```python
from build123d import *

# Parameters (mm, degrees)
SKETCH1_W           = 38.1
SKETCH1_H           = 300
BOSS_EXTRUDE1_DEPTH = 5
SKETCH4_W           = 9
SKETCH4_H           = 40
BOSS_EXTRUDE3_DEPTH = 40
CUT_EXTRUDE2_DEPTH  = 40


with BuildPart() as part:
    # Sketch1 → Boss-Extrude1 (new body)
    with BuildSketch(Plane.XY):
        with BuildLine():
            Line((-30, 275), (-30, 270))
            Line((-30, 270), (-25.725428583, 274.274571417))
            ThreePointArc((-25.725428583, 274.274571417), (-25.725428583, 277.642167462), (-22.357832538, 277.642167462))
            Line((-22.357832538, 277.642167462), (-8.047759053, 291.952240947))
            ThreePointArc((-8.047759053, 291.952240947), (-8.047759053, 295.319836992), (-4.680163008, 295.319836992))
            Line((-4.680163008, 295.319836992), (0, 300))
            Line((0, 300), (-5, 300))
            Line((-5, 300), (-30, 275))
        make_face()
        with BuildLine():
            Line((-25.725428583, 274.274571417), (-30, 270))
            Line((-30, 270), (0, 270))
            Line((0, 270), (0, 300))
            Line((0, 300), (-4.680163008, 295.319836992))
            ThreePointArc((-4.680163008, 295.319836992), (-4.163972894, 294.547303893), (-3.982711031, 293.636038969))
            ThreePointArc((-3.982711031, 293.636038969), (-5.452696107, 291.436050833), (-8.047759053, 291.952240947))
            Line((-8.047759053, 291.952240947), (-22.357832538, 277.642167462))
            ThreePointArc((-22.357832538, 277.642167462), (-21.841642424, 276.869634363), (-21.66038056, 275.95836944))
            ThreePointArc((-21.66038056, 275.95836944), (-23.130365637, 273.758381303), (-25.725428583, 274.274571417))
        make_face()
        with Locations((19.05, 150)):
            Rectangle(SKETCH1_W, SKETCH1_H)
    extrude(amount=BOSS_EXTRUDE1_DEPTH)

    # Sketch4 → Boss-Extrude3 (add)
    with BuildSketch(Plane(origin=(0, 0, 0), x_dir=(-1, 0, 0), z_dir=(0, 0, -1))):
        with Locations((-33.6, 20)):
            Rectangle(SKETCH4_W, SKETCH4_H)
        with Locations((-4.5, 20)):
            Rectangle(SKETCH4_W, SKETCH4_H)
    extrude(amount=BOSS_EXTRUDE3_DEPTH)

    # Sketch5 → Cut-Extrude2 (cut)
    with BuildSketch(Plane(origin=(38.1, 0, 0), x_dir=(0, 0, -1), z_dir=(1, 0, 0))):
        with BuildLine():
            Line((40, 20.01), (40, 40))
            Line((40, 40), (34.145064556, 34.145064556))
            ThreePointArc((34.145064556, 34.145064556), (38.478351855, 27.659841813), (40, 20.01))
        make_face()
        with BuildLine():
            Line((34.145064556, 34.145064556), (40, 40))
            Line((40, 40), (20.01, 40))
            ThreePointArc((20.01, 40), (27.659841813, 38.478351855), (34.145064556, 34.145064556))
        make_face()
        with BuildLine():
            ThreePointArc((26.35, 20), (25.866635031, 22.430039796), (24.490128061, 24.490128061))
            Line((24.490128061, 24.490128061), (15.509871939, 15.509871939))
            ThreePointArc((15.509871939, 15.509871939), (22.430039796, 14.133364969), (26.35, 20))
        make_face()
        with BuildLine():
            Line((15.509871939, 15.509871939), (24.490128061, 24.490128061))
            ThreePointArc((24.490128061, 24.490128061), (15.509871939, 24.490128061), (15.509871939, 15.509871939))
        make_face()
        with BuildLine():
            Line((40, 0), (40, 19.99))
            ThreePointArc((40, 19.99), (34.145064556, 5.854935444), (20.01, 0))
            Line((20.01, 0), (40, 0))
        make_face()
    extrude(amount=-CUT_EXTRUDE2_DEPTH, mode=Mode.SUBTRACT)


solid = part.part
```
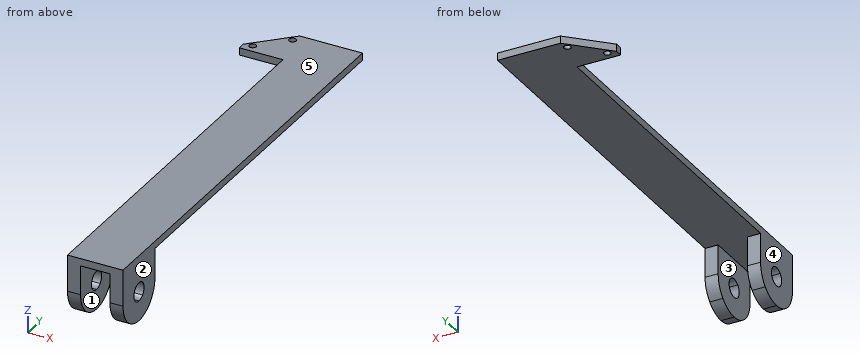
Read the model definition and answer for the solid it produces. Units are mm, in the model's axes. Face numbers are marked on the shaded views. A direction names the side the tool comes from. Give positions to 0.01 mm unless a question says otherwise; leave off trailing zeros. Order: outer loops, then holes, each group sorted by start corner. A loop starts at its lowest first (then second) coordinate and runs counter-clockwise, first axis right, second up.
(1) Straight lines are drawn through the part: L1, parallel to Z at x = 20, y = 92; L2, parallel to X at y = 232, z = 2.5; L3, parallel to Z at x = 33, y = 34. For each, find the intervals that lie inside material, in ascending order.
(2) For the marked faces 1 and 2, determine the directions among +Z, -Z, +X, -X, +Y, -Y from which every point of the face is accessible in a straight line to the end or side of a thin tool.
(3) Find section A-A (x = -14.5). Give the vertices of the cut face in (y, z).
(4) Given pin 1 (4 mm diameter, centred on x = -13.5, z = 2.5, fed in from -Y); pin 2 (20 mm diameter, centred on y = 21, z = -15.5, fed in from -X); pin 3 (12 mm diameter, centred on x = -3.5, y = 52, fed in from -Z); pin 4 (2 mm diameter, centred on x = -15, z = -2, fed in from +Y), each flat-ended and moving along its own axis, determine where each tip first touches the part or whether it passes through.
(5) For a pull along X with two mould halves and no side action, classify the marked faces 3, 4 and 5 as released by +X, released by -X, zero draft, split by the parting line, or undercut.
(6) Find section B-B (y = 84.5). Give the vertices of the cut face in (x, z), plus the area to 4 significant figures.
Result sheet:
1. L1: z = 0 to 5
1. L2: x = 0 to 38.1
1. L3: z = -34.29 to 5
2. face 1: -Z, +Y, -Y
2. face 2: +Z, -Z, +X, +Y, -Y
3. outline: (270, 0) - (290.5, 0) - (290.5, 5) - (270, 5) - close
4. pin 1: stops at y = 270
4. pin 2: stops at x = 0
4. pin 3: stops at z = 0
4. pin 4: passes through
5. face 3: undercut
5. face 4: released by -X
5. face 5: zero draft
6. outline: (0, 0) - (38.1, 0) - (38.1, 5) - (0, 5) - close
6. area: 190.5 mm2
